```python
from build123d import *

# Parameters (mm, degrees)
EXTRUDE_1_DEPTH     = 470
FILLET_1_R          = 7
EXTRUDE_1_2_DEPTH   = 23
SKETCH_5_W          = 14
SKETCH_5_H          = 7
EXTRUDE_2_DEPTH     = 1
FILLET_2_R          = 2
SKETCH_3_R          = 2.5
CUT_EXTRUDE_1_DEPTH = 471.728424891


with BuildPart() as part:
    # Эскиз1 → Extrude 1 (new body)
    with BuildSketch(Plane(origin=(0, 0, 0), x_dir=(1, 0, 0), z_dir=(0, 1, 0))):
        with BuildLine():
            Line((11, -11.5), (11, 7.5))
            ThreePointArc((11, 7.5), (9.828427125, 10.328427125), (7, 11.5))
            Line((7, 11.5), (-7, 11.5))
            ThreePointArc((-7, 11.5), (-9.828427125, 10.328427125), (-11, 7.5))
            Line((-11, 7.5), (-11, -11.5))
            Line((-11, -11.5), (-10, -11.5))
            Line((-10, -11.5), (-10, 7.5))
            ThreePointArc((-10, 7.5), (-9.121320344, 9.621320344), (-7, 10.5))
            Line((-7, 10.5), (7, 10.5))
            ThreePointArc((7, 10.5), (9.121320344, 9.621320344), (10, 7.5))
            Line((10, 7.5), (10, -11.5))
            Line((10, -11.5), (11, -11.5))
        make_face()
    extrude(amount=EXTRUDE_1_DEPTH)

    # Скругление1
    fillet_1_edges = [part.edges().sort_by_distance(p)[0] for p in [
        (-10.5, 0, 11.5),
        (10.5, 0, 11.5),
    ]]
    fillet(fillet_1_edges, radius=FILLET_1_R)

    # Эскиз2 → Extrude 1 2 (add)
    with BuildSketch(Plane(origin=(0, 470, 0), x_dir=(1, 0, 0), z_dir=(0, 1, 0))):
        with BuildLine():
            Line((-12, -11.5), (-12, 7.5))
            ThreePointArc((-12, 7.5), (-10.535533906, 11.035533906), (-7, 12.5))
            Line((-7, 12.5), (7, 12.5))
            ThreePointArc((7, 12.5), (10.535533906, 11.035533906), (12, 7.5))
            Line((12, 7.5), (12, -11.5))
            Line((12, -11.5), (12, -12))
            Line((12, -12), (-12, -12))
            Line((-12, -12), (-12, -11.5))
        make_face()
    extrude(amount=-EXTRUDE_1_2_DEPTH)

    # Эскиз5 → Бобышка-Вытянуть2 (add)
    with BuildSketch(Plane(origin=(0, 0, -11.5), x_dir=(-1, 0, 0), z_dir=(0, 0, -1))):
        with Locations((0, -3.5)):
            Rectangle(SKETCH_5_W, SKETCH_5_H)
    extrude(amount=-EXTRUDE_2_DEPTH)

    # Скругление2
    fillet_2_edges = [part.edges().sort_by_distance(p)[0] for p in [
        (7, -7, -11),
        (-7, -7, -11),
    ]]
    fillet(fillet_2_edges, radius=FILLET_2_R)

    # Эскиз3 → Вырез-Вытянуть1 (cut, through all)
    with BuildSketch(Plane.ZY.offset(11)):
        with Locations((2.5, 9)):
            Circle(SKETCH_3_R)
        with Locations((2.5, 224)):
            Circle(SKETCH_3_R)
    extrude(amount=-CUT_EXTRUDE_1_DEPTH, mode=Mode.SUBTRACT)


solid = part.part
```
Build history of the part. All positions in model axes, mm. A direction names the side the tool comes from. Round coordinates to 2 decimals unless told otherwise and drop trailing zeros. Order: outer loops, then holes, each group sorted by start corner. A loop starts at its lowest first (then second) coordinate and runs counter-clockwise, first axis right, second up. Notation, with made-up numbers: (42, 52) -> (66, 52) arc R17 cw to (66, 77) -> close; hole circle Ø3 at (41.25, 65.25). An arc over 180 degrees is marked (long way). Answer in a Markdown table with one row per item.
1) Wall check: L1, parallel to Y at x = 10.75, z = 2.5; L2, parallel to X at y = 337, z = 10; L3, parallel to Z at x = 6.75, y = 320. Give the ranges that are in metal, low to high.
Values:
| item | result |
|---|---|
| L1 | 0 to 6.5, 11.5 to 221.5, 226.5 to 470 |
| L2 | -11 to -10, 10 to 11 |
| L3 | -11.5 to -10.5 |
2) Pin check, flat tips, straight feed: P1, Ø1.5, axis at x = -2.5, z = -5, coming from the -Y side; P2, Ø1.5, axis at x = 4, y = 312, coming from the +Z side; P3, Ø5.5, axis at y = 286.5, z = 4, coming from the -X side. Stop position of each tip, or through.
Values:
| item | result |
|---|---|
| P1 | y = 447 |
| P2 | z = -10.5 |
| P3 | x = -11 |
3) Which spindle directions (+Z, -Z, +X, -X, +Y, -Y) get a long thin tool onto all of the face, cutting with end or side? Do faces 1 (the flat face through (-11, 220, 2)), 2 (the flat face through (0, 223, -10.5)), 3 (the flat face through (0, 223, -11.5)). Say none if no direction does.
Values:
| item | result |
|---|---|
| face 1 | +Z, -Z, -X, -Y |
| face 2 | +Z, -Y |
| face 3 | -Z, +X, -X, -Y |
4) Mould opens along X. For faces 4 (the flat face through (-12, 459, 2)), 5 (the flat face through (10, 220, 2)), 6 (the flat face through (0, 459, -12.5)), 7 (the flat face through (11, 220, 2)) say: released by +X, released by -X, zero draft, split by the parting line, or undercut.
Values:
| item | result |
|---|---|
| face 4 | released by -X |
| face 5 | undercut |
| face 6 | zero draft |
| face 7 | released by +X |
5) Band-saw the part on A-A on y = 291. Give the cut face in (x, z).
Values:
| item | result |
|---|---|
| outline | (-11, -7.5) arc R4 ccw to (-7, -11.5) -> (7, -11.5) arc R4 ccw to (11, -7.5) -> (11, 11.5) -> (10, 11.5) -> (10, -7.5) arc R3 cw to (7, -10.5) -> (-7, -10.5) arc R3 cw to (-10, -7.5) -> (-10, 11.5) -> (-11, 11.5) -> close |
